from build123d import *

# Parameters (mm, degrees)
BOSS_EXTRUDE1_DEPTH            = 13
SKETCH2_W                      = 9
SKETCH2_H                      = 12
CUT_EXTRUDE1_DEPTH             = 5
SKETCH3_R                      = 1.1
SKETCH3_R_2                    = 1.2
CUT_EXTRUDE2_DEPTH             = 5
SKETCH4_R                      = 1.5
BOSS_EXTRUDE3_DEPTH            = 3
BOSS_EXTRUDE4_START            = -6
BOSS_EXTRUDE4_OUTLINE_R        = 1.5
BOSS_EXTRUDE4_DEPTH            = 3
CUT_EXTRUDE3_REACH             = 53.746
SKETCH9_R                      = 1.5
CUT_EXTRUDE3_DIRECTION_2_DEPTH = 52.745889594
SKETCH10_W                     = 1
SKETCH10_H                     = 15.6
CUT_EXTRUDE5_DEPTH             = 39.790984582


# Read off the part's stored shape, not the designer's step: Boss-Extrude4
with BuildPart() as part:
    # Sketch1 → Boss-Extrude1 (new body)
    with BuildSketch(Plane.XY):
        Polygon((-11.5, 0), (11.5, 0), (16.5, 0), (16.5, 20.6), (11.5, 20.6), (11.5, 5), (-11.5, 5), (-11.5, 20.6), (-16.5, 20.6), (-16.5, 0), align=None)
    extrude(amount=BOSS_EXTRUDE1_DEPTH)

    # Sketch2 → Cut-Extrude1 (cut)
    with BuildSketch(Plane(origin=(-11.5, 0, 0), x_dir=(0, 0, -1), z_dir=(1, 0, 0))):
        with Locations((-8.5, 11)):
            Rectangle(SKETCH2_W, SKETCH2_H)
    extrude(amount=-CUT_EXTRUDE1_DEPTH, mode=Mode.SUBTRACT)

    # Sketch3 → Cut-Extrude2 (cut)
    with BuildSketch(Plane(origin=(0, 20.6, 0), x_dir=(1, 0, 0), z_dir=(0, 1, 0))):
        with Locations(Location((-13.63, -6.2, 0), (0, 0, 180))):
            Circle(SKETCH3_R)
        with Locations((14.132964109, -6.2)):
            Circle(SKETCH3_R_2)
    extrude(amount=-CUT_EXTRUDE2_DEPTH, mode=Mode.SUBTRACT)

    # Sketch4 → Boss-Extrude3 (add)
    with BuildSketch(Plane.XY.offset(13)):
        with BuildLine():
            Line((22.42265834, 22.604489903), (16.5, 20.6))
            Line((16.5, 20.6), (16.5, 16.600005885))
            Line((16.5, 16.600005885), (24.538834173, 19.320695429))
            ThreePointArc((24.538834173, 19.320695429), (26.893762727, 23.162043036), (22.42265834, 22.604489903))
        make_face()
        with Locations((24.792321364, 21.807811077)):
            Circle(SKETCH4_R, mode=Mode.SUBTRACT)
    extrude(amount=-BOSS_EXTRUDE3_DEPTH)

    # Boss-Extrude4 outline → Boss-Extrude4 (add)
    with BuildSketch(Plane(origin=(0, 0, 0), x_dir=(-1, 0, 0), z_dir=(0, 0, -1)).offset(BOSS_EXTRUDE4_START)):
        with BuildLine():
            Line((-16.499998213, 20.600005281), (-22.42265834, 22.604489903))
            ThreePointArc((-22.42265834, 22.604489903), (-26.893762727, 23.162043036), (-24.538834173, 19.320695429))
            Line((-24.538834173, 19.320695429), (-16.5, 16.600005885))
            Line((-16.5, 16.600005885), (-16.499998213, 20.600005281))
        make_face()
        with Locations((-24.792321364, 21.807811077)):
            Circle(BOSS_EXTRUDE4_OUTLINE_R, mode=Mode.SUBTRACT)
    extrude(amount=BOSS_EXTRUDE4_DEPTH)

    # Sketch9 → Cut-Extrude3 (cut, up to next)
    with BuildSketch(Plane.ZY.offset(16.5), mode=Mode.PRIVATE) as cut_extrude3_sk1:
        with Locations(Location((2.5, 18.8, 0), (0, 0, 90))):
            Circle(SKETCH9_R)
    cut_extrude3_tool1 = extrude(cut_extrude3_sk1.sketch, amount=-CUT_EXTRUDE3_REACH, mode=Mode.PRIVATE) & part.part
    # Sketch9 → Cut-Extrude3 (cut, up to next)
    with BuildSketch(Plane.ZY.offset(16.5), mode=Mode.PRIVATE) as cut_extrude3_sk2:
        with Locations(Location((10.5, 18.8, 0), (0, 0, 90))):
            Circle(SKETCH9_R)
    cut_extrude3_tool2 = extrude(cut_extrude3_sk2.sketch, amount=-CUT_EXTRUDE3_REACH, mode=Mode.PRIVATE) & part.part
    add(cut_extrude3_tool1.solids().sort_by_distance((-16.5, 18.8, 2.5))[0], mode=Mode.SUBTRACT)
    add(cut_extrude3_tool2.solids().sort_by_distance((-16.5, 18.8, 10.5))[0], mode=Mode.SUBTRACT)

    # Sketch9 → Cut-Extrude3 direction 2 (cut)
    with BuildSketch(Plane.ZY.offset(16.5)):
        with Locations(Location((2.5, 18.8, 0), (0, 0, 90))):
            Circle(SKETCH9_R)
        with Locations(Location((10.5, 18.8, 0), (0, 0, 90))):
            Circle(SKETCH9_R)
    extrude(amount=CUT_EXTRUDE3_DIRECTION_2_DEPTH, mode=Mode.SUBTRACT)

    # Sketch10 → Cut-Extrude5 (cut, through all)
    with BuildSketch(Plane.XY.offset(13)):
        with Locations((-12, 12.8)):
            Rectangle(SKETCH10_W, SKETCH10_H)
    extrude(amount=-CUT_EXTRUDE5_DEPTH, mode=Mode.SUBTRACT)


solid = part.part
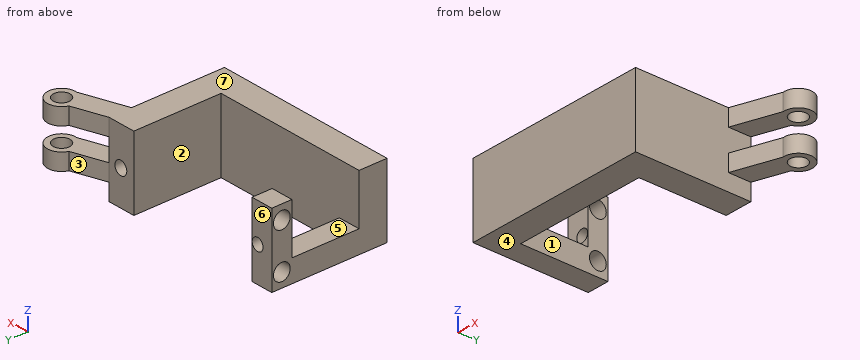
Work out the finished part from the listing and answer in its coordinate system (mm). Face numbers are marked on the shaded views. A direction names the side the tool comes from. Coordinates: 2 decimals unless noted, no trailing zeros. Loops run counter-clockwise (first coordinate to the right, second up) from the corner with the lowest first, then second, coordinate; pieces in that order, holes last. Notation, with made-up numbers: (43, 40.5) -> (56, 40.5) arc R24 cw to (56, 67.5) -> close; hole circle Ø11 at (-23.75, -13). An arc over 180 degrees is marked (long way). Write each question's results on one line, items separated by ' | '. Start each with the question number.
1) Consider line 1 along Z through (x, y) = (-13.65, 18.8); line 2 along X through (y, z) = (9.75, 3.25); line 3 along Y through (x, z) = (-7, 5). Determine where each line is inside the solid, lowest interval first.
2) Find section C-C on y = 18.8. Determine the outline of the cut face in (x, z), then the cut area to 3 significant figures.
3) Flat-ended cylindrical pins translate along their axes: P1, Ø2, axis at x = -3, z = 7.5, coming from the +Y side; P2, Ø2, axis at x = -14, y = 10.5, coming from the +Z side; P3, Ø2.5, axis at x = 24.79, y = 21.81, coming from the -Z side; P4, Ø1.2, axis at x = -15, z = 5, coming from the +Y side. Find the tip coordinate at first contact, or state that the pin passes through.
4) Find section B-B on z = 10.5. Determine the outline of the cut face in (x, y).
5) The mould has two halves that part along X. Classify the marked faces 1, 2, 3 and 4: pulls with the +X half, pulls with the -X half, needs draft (parallel to the pull), parting line crosses it, or undercut.
6) For the marked faces 5, 6 and 7, determine the directions among +Z, -Z, +X, -X, +Y, -Y from which every point of the face is accessible in a straight line to the end or side of a thin tool.
7) Find section D-D on z = 2.5. Determine the outline of the cut face in (x, y).
8) Find section A-A on x = -13.63. Determine the outline of the cut face in (y, z), then the cut area to 3 significant figures.
Response values:
1) line 1: z = 0 to 1, 4 to 5.1, 7.3 to 9, 12 to 13 | line 2: x = -16.5 to -12.5, 11.5 to 16.5 | line 3: y = 0 to 5
2) outline: (-16.5, 0) -> (-12.5, 0) -> (-12.5, 1) -> (-16.5, 1) -> close; (-16.5, 4) -> (-12.5, 4) -> (-12.5, 9) -> (-16.5, 9) -> close; (-16.5, 12) -> (-12.5, 12) -> (-12.5, 13) -> (-16.5, 13) -> close; (11.5, 0) -> (16.5, 0) -> (16.5, 3) -> (23, 3) -> (23, 6) -> (16.5, 6) -> (16.5, 10) -> (23, 10) -> (23, 13) -> (11.5, 13) -> close; hole circle Ø2.2 at (-13.63, 6.2); hole circle Ø2.4 at (14.13, 6.2) | area: 124 mm^2
3) P1: stops at y = 5 | P2: stops at z = 4 | P3: passes through | P4: stops at y = 20.6
4) outline: (-16.5, 0) -> (16.5, 0) -> (16.5, 16.6) -> (24.54, 19.32) arc R2.5 ccw (long way) to (22.42, 22.6) -> (16.5, 20.6) -> (11.5, 20.6) -> (11.5, 5) -> (-16.5, 5) -> close; (-16.5, 17) -> (-12.5, 17) -> (-12.5, 17.3) -> (-16.5, 17.3) -> close; (-16.5, 20.3) -> (-12.5, 20.3) -> (-12.5, 20.6) -> (-16.5, 20.6) -> close; hole circle Ø3 at (24.79, 21.81)
5) face 1: undercut | face 2: undercut | face 3: pulls with the -X half | face 4: needs draft
6) face 5: +Z, -X | face 6: +Z, -Z, -X, +Y | face 7: +Z, +X, -X, +Y, -Y
7) outline: (-16.5, 0) -> (16.5, 0) -> (16.5, 20.6) -> (11.5, 20.6) -> (11.5, 5) -> (-12.5, 5) -> (-12.5, 17.3) -> (-16.5, 17.3) -> close; (-16.5, 20.3) -> (-12.5, 20.3) -> (-12.5, 20.6) -> (-16.5, 20.6) -> close
8) outline: (0, 0) -> (20.6, 0) -> (20.6, 5.1) -> (17, 5.1) -> (17, 4) -> (5, 4) -> (5, 13) -> (0, 13) -> close; (17, 7.3) -> (20.6, 7.3) -> (20.6, 13) -> (17, 13) -> close; hole circle Ø3 at (18.8, 2.5); hole circle Ø3 at (18.8, 10.5) | area: 138 mm^2
